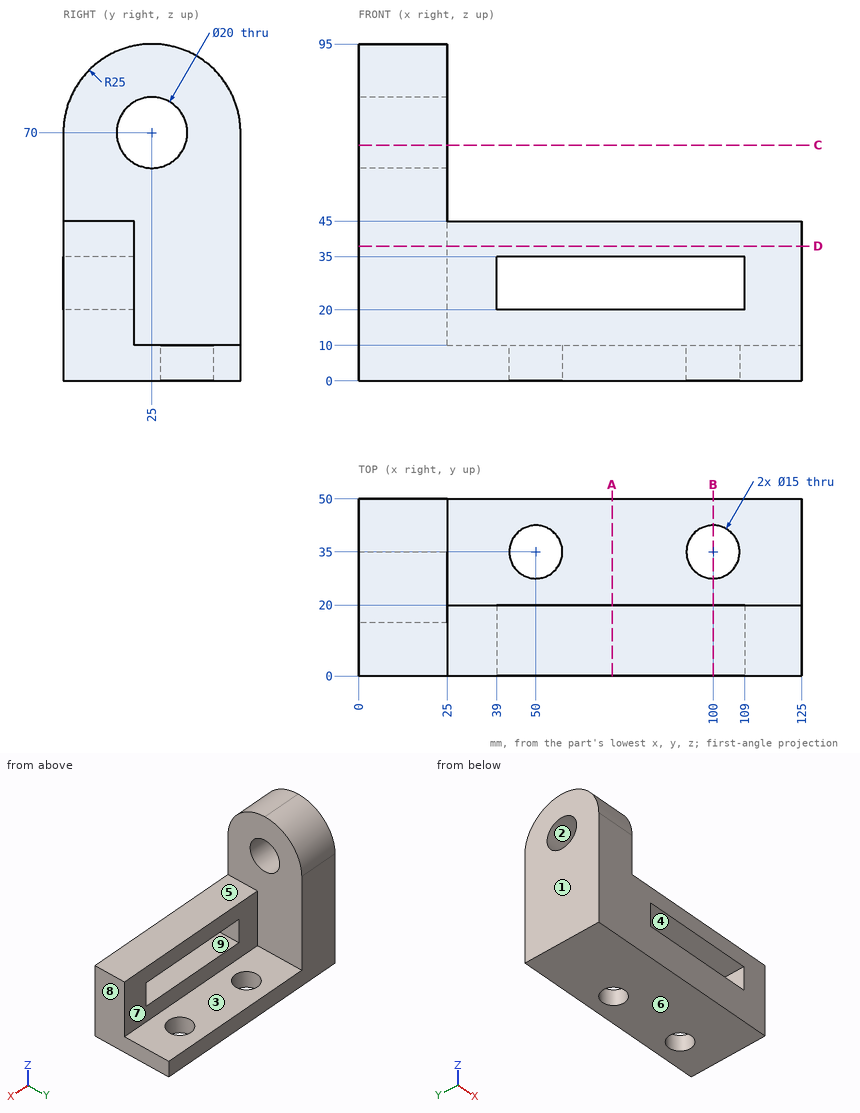
Verification items for this drawing (mm, ordinates from the low corner). A direction names the side the tool comes from. Give positions to 0.01 mm unless a question says otherwise; leave off trailing zeros. Write each loop counter-clockwise with the first axis right and the second up, starting at its lowest first coordinate (ties: lowest second). Pieces come first, ordered by that corner, then holes. Notation, with made-up numbers: (24.25, -33.75) - (58.25, -33.75) arc R19 ccw to (58.25, -20.75) - close; hole circle Ø2 at (14, 45). An arc over 180 degrees is marked (long way). Answer as CSV lines item,"result". Start each with the question number.
1. Sectioned sample at D-D (z = 38). Record the boundary of the cut face in (x, y), then the cut area to 3 significant figures.
2. Draft check along Z on the marked faces 1, 2, 3 and 4. Enter one of: pulls with the +Z half, pulls with the -Z half, needs draft (parallel to the pull), parting line crosses it, or undercut.
3. Set-up check for the marked faces 5, 6, 7, 8 and 9: record each of +Z, -Z, +X, -X, +Y, -Y from which the full face is reachable in a straight line by a thin tool's end or side.
4. Sectioned sample at A-A (x = 71.5). Record the boundary of the cut face in (y, z), then the cut area to 3 significant figures.
5. Thickness scan on line 1 (Z direction, x = 50.5, y = 17.5); line 2 (Y direction, x = 50, z = 7); line 3 (X direction, y = 24, z = 13). Record the ranges inside material, lowest first.
6. Sectioned sample at B-B (x = 100). Record the boundary of the cut face in (y, z), then the cut area to 3 significant figures.
7. Depth check by flat-ended pin: pin 1 (9 mm diameter, centred on x = 100, y = 35, fed in from -Z); pin 2 (22 mm diameter, centred on x = 91.5, y = 14, fed in from +Z); pin 3 (5 mm diameter, centred on x = 63, z = 40, fed in from +Y); pin 4 (4 mm diameter, centred on x = 106.5, y = 31.5, fed in from +Z). Enter the tip coordinate at first touch or a pass-through.
8. Sectioned sample at C-C (z = 66.5). Record the boundary of the cut face in (x, y).
Derived:
1,outline,"(0, 0) - (125, 0) - (125, 20) - (25, 20) - (25, 50) - (0, 50) - close"
1,area,"3,250 mm²"
2,face 1,"needs draft"
2,face 2,"undercut"
2,face 3,"pulls with the +Z half"
2,face 4,"undercut"
3,face 5,"+Z, +X, +Y, -Y"
3,face 6,"-Z, +X, -X, +Y, -Y"
3,face 7,"+Z, +X, +Y"
3,face 8,"+Z, -Z, +X, +Y, -Y"
3,face 9,"+Y, -Y"
4,outline,"(0, 0) - (50, 0) - (50, 10) - (20, 10) - (20, 20) - (0, 20) - close; (0, 35) - (20, 35) - (20, 45) - (0, 45) - close"
4,area,"900 mm²"
5,line 1,"0 to 20, 35 to 45"
5,line 2,"0 to 27.5, 42.5 to 50"
5,line 3,"0 to 25"
6,outline,"(0, 0) - (27.5, 0) - (27.5, 10) - (20, 10) - (20, 20) - (0, 20) - close; (0, 35) - (20, 35) - (20, 45) - (0, 45) - close; (42.5, 0) - (50, 0) - (50, 10) - (42.5, 10) - close"
6,area,"750 mm²"
7,pin 1,"through"
7,pin 2,"z = 45"
7,pin 3,"y = 20"
7,pin 4,"z = 10"
8,outline,"(0, 0) - (25, 0) - (25, 15.63) - (0, 15.63) - close; (0, 34.37) - (25, 34.37) - (25, 50) - (0, 50) - close"
